Build history of the part. All positions in model axes, mm. Face numbers are marked on the shaded views. A direction names the side the tool comes from. Give positions to 0.01 mm unless a question says otherwise; leave off trailing zeros. Write each loop counter-clockwise with the first axis right and the second up, starting at its lowest first coordinate (ties: lowest second). Pieces come first, ordered by that corner, then holes. Notation, with made-up numbers: M 12.5,67.25 L 18.5,67.25 A8 ccw 18.5,81.25 Z; hole C 66,19.5 d3. An arc over 180 degrees is marked long. One line per item, written item: value. Start each with the question number.
Autodesk Inventor part; units mm, degrees
ref_plane "YZ Plane" through (0, 0, 0) normal (1, 0, 0) x (0, 1, 0)
ref_plane "XZ Plane" through (0, 0, 0) normal (0, 1, 0) x (-1, 0, 0)
ref_plane "XY Plane" through (0, 0, 0) normal (0, 0, 1) x (1, 0, 0)
sketch "Sketch1" plane through (0, 0, 0) normal (0, 0, 1) x (1, 0, 0)
  line L0 (51, -45) -> (-51, -45)
  line L1 (-51, -45) -> (-51, 45)
  line L2 (-51, 45) -> (51, 45)
  line L3 (51, 45) -> (51, -45)
  line L4 (51, -45) -> (-51, 45) construction
  line L5 (-51, -45) -> (51, 45) construction
  line L6 (-22, 0) -> (22, 0) construction
  line L7 (-36, 35) -> (-8, 35)
  line L8 (-8, 35) -> (-8, -35)
  line L9 (-8, -35) -> (-36, -35)
  line L10 (-36, -35) -> (-36, 35)
  line L11 (-36, 35) -> (-8, -35) construction
  line L12 (-8, 35) -> (-36, -35) construction
  line L13 (36, 35) -> (8, 35)
  line L14 (8, 35) -> (8, -35)
  line L15 (8, -35) -> (36, -35)
  line L16 (36, -35) -> (36, 35)
  line L17 (36, 35) -> (8, -35) construction
  line L18 (8, 35) -> (36, -35) construction
  point P0 (0, 0)
  point P1 (0, 0)
  dimension "d0" = 16
  dimension "d1" = 28
  dimension "d2" = 28
  dimension "d3" = 70
  dimension "d4" = 10
  dimension "d5" = 15
extrude "Extrusion1" add sketch "Sketch1" along normal blind 15
sketch "Sketch2" plane through (51, -45, 0) normal (1, 0, 0) x (0, 0, -1)
  circle A0 centre (0, 45) radius 5
  point P0 (0, 45)
  dimension "d8" = 10
extrude "Extrusion2" cut sketch "Sketch2" against normal through all
sketch "Sketch3" plane through (51, -45, 15) normal (1, 0, 0) x (0, 0, -1)
  arc A0 (15, 50) -> (15, 40) centre (15, 45) ccw
  circle A1 centre (15, 45) radius 11
  dimension "d11" = 22
extrude "Extrusion3" cut sketch "Sketch3" against normal blind 7
sketch "Sketch4" plane through (-51, -45, 15) normal (-1, 0, 0) x (0, 0, 1)
  arc A0 (-15, 40) -> (-15, 50) centre (-15, 45) ccw
  circle A1 centre (-15, 45) radius 11
  dimension "d14" = 22
extrude "Extrusion4" cut sketch "Sketch4" against normal blind 7
sketch "Sketch5" plane through (-8, -35, 15) normal (-1, 0, 0) x (0, 0, 1)
  arc A0 (-15, 30) -> (-15, 40) centre (-15, 35) ccw
  circle A1 centre (-15, 35) radius 11
  dimension "d17" = 22
extrude "Extrusion5" cut sketch "Sketch5" against normal blind 7
sketch "Sketch6" plane through (8, -35, 15) normal (1, 0, 0) x (0, 0, -1)
  arc A0 (15, 40) -> (15, 30) centre (15, 35) ccw
  circle A1 centre (15, 35) radius 11
  dimension "d20" = 22
extrude "Extrusion6" cut sketch "Sketch6" against normal blind 7
sketch "Sketch7" plane through (0, 0, 15) normal (0, 0, 1) x (1, 0, 0)
  line L0 (-36, -35) -> (-36, 35)
  line L1 (-51, 45) -> (-51, -45)
  line L2 (0, 30) -> (0, -30) construction
  circle A0 centre (0, 30) radius 4
  circle A1 centre (0, -30) radius 4
  line L3 (43.5, -30) -> (-43.5, -30) construction
  line L4 (-43.5, -30) -> (-43.5, 30) construction
  line L5 (-43.5, 30) -> (43.5, 30) construction
  line L6 (43.5, 30) -> (43.5, -30) construction
  line L7 (43.5, -30) -> (-43.5, 30) construction
  line L8 (-43.5, -30) -> (43.5, 30) construction
  circle A2 centre (-43.5, 30) radius 4
  circle A3 centre (-43.5, -30) radius 4
  circle A4 centre (43.5, -30) radius 4
  circle A5 centre (43.5, 30) radius 4
  point P0 (0, 0)
  point P1 (0, 0)
  dimension "d23" = 60
  dimension "d24" = 8
  dimension "d25" = 7.5
  dimension "d26" = 87
extrude "Extrusion7" cut sketch "Sketch7" against normal through all
sketch "Sketch8" plane through (0, 0, 15) normal (0, 0, 1) x (1, 0, 0)
  line L0 (-51, 45) -> (-86, 45)
  line L1 (-86, 45) -> (-86, 31)
  line L2 (-86, 31) -> (-51, 31)
  line L3 (-51, 31) -> (-51, 45)
  line L4 (-51, -45) -> (-86, -45)
  line L5 (-86, -45) -> (-86, -31)
  line L6 (-86, -31) -> (-51, -31)
  line L7 (-51, -31) -> (-51, -45)
  line L8 (-86, 45) -> (-101, 45)
  line L9 (-101, 45) -> (-101, -45)
  line L10 (-101, -45) -> (-86, -45)
  line L11 (-86, -45) -> (-86, 45)
  point P0 (0, 0)
  dimension "d29" = 14
  dimension "d30" = 15
  dimension "d31" = 35
extrude "Extrusion8" add sketch "Sketch8" against normal up to surface (15 mm away)
sketch "Sketch9" plane through (-101, -45, 15) normal (-1, 0, 0) x (0, 0, 1)
  circle A0 centre (-15, 45) radius 11
  dimension "d34" = 22
extrude "Extrusion9" cut sketch "Sketch9" against normal up to surface (50 mm away)
sketch "Sketch10" plane through (0, 0, 0) normal (0, 0, -1) x (-1, 0, 0)
  line L0 (101, -11) -> (86, -11)
  circle A0 centre (43.5, 30) radius 4
  circle A1 centre (0, 30) radius 4
  circle A2 centre (-43.5, 30) radius 4
  line L1 (86, 11) -> (101, 11)
  line L2 (101, 11) -> (101, 45)
  line L3 (101, 45) -> (-51, 45)
  line L4 (-51, 45) -> (-51, 11)
  line L5 (-51, 11) -> (-44, 11)
  line L6 (-44, 11) -> (-44, 5)
  line L7 (-44, 5) -> (-36, 5)
  line L8 (-36, 5) -> (-36, 35)
  line L9 (-36, 35) -> (-8, 35)
  line L10 (-8, 35) -> (-8, 11)
  line L11 (-8, 11) -> (-1, 11)
  line L12 (-1, 11) -> (-1, 5)
  line L13 (-1, 5) -> (1, 5)
  line L14 (1, 5) -> (1, 11)
  line L15 (1, 11) -> (8, 11)
  line L16 (8, 11) -> (8, 35)
  line L17 (8, 35) -> (36, 35)
  line L18 (36, 35) -> (36, 5)
  line L19 (36, 5) -> (44, 5)
  line L20 (44, 5) -> (44, 11)
  line L21 (44, 11) -> (51, 11)
  line L22 (51, 11) -> (51, 31)
  line L23 (51, 31) -> (86, 31)
  line L24 (86, 31) -> (86, 11)
  line L25 (93.5, 11) -> (93.5, 21) construction
  line L26 (93.5, -11) -> (93.5, -21) construction
  circle A3 centre (93.5, 21) radius 4
  circle A4 centre (93.5, -21) radius 4
  point P0 (0, 0)
  dimension "d37" = 8
  dimension "d38" = 10
extrude "Extrusion10" cut sketch "Sketch10" against normal through all contours A3 | A4
properties part number "frame 1"
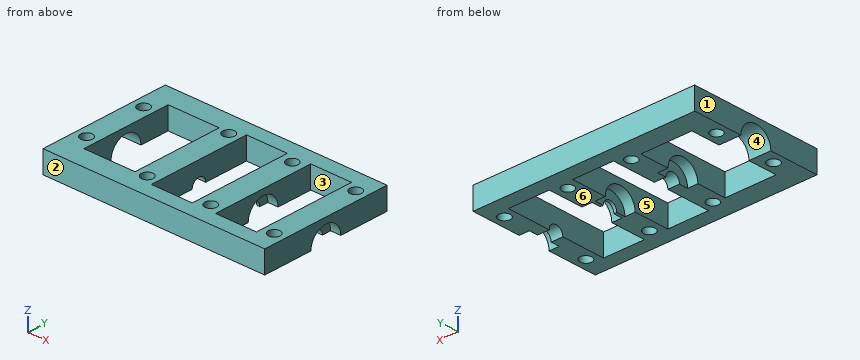
1) Band-saw the part on B-B (y = 0). List the corners of the cut face in (x, z).
2) Tool access for the marked faces 4, 5 and 6: list every direction of +Z, -Z, +X, -X, +Y, -Y with a clear straight run to the whole face (end or side of a thin tool).
3) Band-saw the part on C-C (y = 21). List the corners of the cut face in (x, z), then the cut area to 3 significant figures.
4) Band-saw the part on D-D (x = -41). List the corners of the cut face in (y, z).
5) Band-saw the part on A-A (x = -82). List the corners of the cut face in (y, z).
6) Drop flat-ended pins along their axis: P1, Ø3.5, axis at y = -2, z = 7, coming from the +X side; P2, Ø3.5, axis at y = -3.5, z = 4.5, coming from the -X side. Give the stop position or say it passes through.
7) Mould opens along Y. For the marked faces 1, 2 and 3 say: released by +Y, released by -Y, zero draft, split by the parting line, or undercut.
8) Probe line 1 along X through (y, z) = (13.5, 3); line 2 along Y through (x, z) = (43.5, 7); line 3 along Y through (x, z) = (-51.5, 13). List the from-to ranges inside material, lowest first. Write a range as from..to.
Model answer:
1. outline: M -101,11 L -86,11 L -86,15 L -101,15 Z; M -51,11 L -44,11 L -44,5 L -36,5 L -36,15 L -51,15 Z; M -8,11 L -1,11 L -1,5 L 1,5 L 1,11 L 8,11 L 8,15 L -8,15 Z; M 36,5 L 44,5 L 44,11 L 51,11 L 51,15 L 36,15 Z
2. face 4: -Z, -X
2. face 5: +Z, -Z
2. face 6: -Z, +X, -X, +Y, -Y
3. outline: M -101,0 L -97.5,0 L -97.5,15 L -101,15 Z; M -89.5,0 L -86,0 L -86,15 L -89.5,15 Z; M -51,0 L -36,0 L -36,15 L -51,15 Z; M -8,0 L 8,0 L 8,15 L -8,15 Z; M 36,0 L 51,0 L 51,15 L 36,15 Z
3. area: 795 mm²
4. outline: M -45,0 L -33.12,0 L -33.12,15 L -45,15 Z; M -26.88,0 L -5,0 A5 cw 5,0 L 26.88,0 L 26.88,15 L -26.88,15 Z; M 33.12,0 L 45,0 L 45,15 L 33.12,15 Z
5. outline: M -45,0 L -31,0 L -31,15 L -45,15 Z; M 31,0 L 45,0 L 45,15 L 31,15 Z
6. P1: stops at x = 44
6. P2: stops at x = -44
7. face 1: zero draft
7. face 2: released by -Y
7. face 3: undercut
8. line 1: x = -101..-86, -51..-36, -8..8, 36..51
8. line 2: y = -45..-34, -26..26, 34..45
8. line 3: y = -45..-31, 31..45
